from build123d import *

# Parameters (mm, degrees)
F0_R     = 3.175
F1_DEPTH = 3.048


with BuildPart() as f1:
    # F0 (on Front) → F1 (new body)
    with BuildSketch(Plane.XZ):
        with BuildLine():
            ThreePointArc((18.5272162363, -2.8907946242), (12.1944256202, -14.2446628188), (0, -18.7513848829))
            Line((0, -18.7513848829), (0, -51.0613519013))
            ThreePointArc((0, -51.0613519013), (6.7351920908, -53.8511598105), (9.525, -60.5863519013))
            Line((9.525, -60.5863519013), (36.5125, -60.5863519013))
            ThreePointArc((36.5125, -60.5863519013), (38.9380895153, -54.8747191174), (44.7324052746, -52.6538772867))
            Line((44.7324052746, -52.6538772867), (19.9038367454, -51.7699515192))
            ThreePointArc((19.9038367454, -51.7699515192), (14.056218392, -48.8866966862), (12.3315367458, -42.5991477155))
            Line((12.3315367458, -42.5991477155), (18.5272162363, -2.8907946242))
        make_face()
        with BuildLine():
            Line((36.5125, -60.5863519013), (9.525, -60.5863519013))
            ThreePointArc((9.525, -60.5863519013), (6.9705567315, -67.0776509895), (0.6773435479, -70.0872376873))
            Line((0.6773435479, -70.0872376873), (44.7324052746, -68.5188265159))
            ThreePointArc((44.7324052746, -68.5188265159), (38.9380895153, -66.2979846852), (36.5125, -60.5863519013))
        make_face()
        with BuildLine():
            Line((0, 18.7513848829), (0, 3.175))
            ThreePointArc((0, 3.175), (2.2450640303, 2.2450640303), (3.175, 0))
            ThreePointArc((3.175, 0), (2.2450640303, -2.2450640303), (0, -3.175))
            Line((0, -3.175), (0, -18.7513848829))
            ThreePointArc((0, -18.7513848829), (12.1944256202, -14.2446628188), (18.5272162363, -2.8907946242))
            ThreePointArc((18.5272162363, -2.8907946242), (18.6952587236, -1.4497366262), (18.7513848829, 0))
            ThreePointArc((18.7513848829, 0), (18.6943609499, 1.4612678406), (18.5236359763, 2.9136480987))
            Line((18.5236359763, 2.9136480987), (18.3973654955, 3.6264828487))
            ThreePointArc((18.3973654955, 3.6264828487), (11.9082504878, 14.4847507865), (0, 18.7513848829))
        make_face()
        with BuildLine():
            ThreePointArc((0, -3.175), (-3.175, 0), (0, 3.175))
            Line((0, 3.175), (0, 18.7513848829))
            ThreePointArc((0, 18.7513848829), (-12.0470149388, 14.3695464817), (-18.4637179825, 3.2719341818))
            ThreePointArc((-18.4637179825, 3.2719341818), (-18.7503896007, 0.1931963966), (-18.5272162363, -2.8907946242))
            ThreePointArc((-18.5272162363, -2.8907946242), (-12.1944256202, -14.2446628188), (0, -18.7513848829))
            Line((0, -18.7513848829), (0, -3.175))
        make_face()
        with BuildLine():
            Line((0, -57.4113519013), (0, -51.0613519013))
            ThreePointArc((0, -51.0613519013), (-6.7351920908, -53.8511598105), (-9.525, -60.5863519013))
            ThreePointArc((-9.525, -60.5863519013), (-6.7351920908, -67.3215439921), (0, -70.1113519013))
            Line((0, -70.1113519013), (0.6773435479, -70.0872376873))
            ThreePointArc((0.6773435479, -70.0872376873), (6.9705567315, -67.0776509895), (9.525, -60.5863519013))
            Line((9.525, -60.5863519013), (3.175, -60.5863519013))
            ThreePointArc((3.175, -60.5863519013), (-2.2450640303, -62.8314159316), (0, -57.4113519013))
        make_face()
        with BuildLine():
            ThreePointArc((9.525, -60.5863519013), (6.7351920908, -53.8511598105), (0, -51.0613519013))
            Line((0, -51.0613519013), (0, -57.4113519013))
            ThreePointArc((0, -57.4113519013), (2.2450640303, -58.341287871), (3.175, -60.5863519013))
            Line((3.175, -60.5863519013), (9.525, -60.5863519013))
        make_face()
        with BuildLine():
            ThreePointArc((-18.4637179825, 3.2719341818), (-12.0470149388, 14.3695464817), (0, 18.7513848829))
            Line((0, 18.7513848829), (0, 36.5252))
            Line((0, 36.5252), (0, 44.1886480987))
            ThreePointArc((0, 44.1886480987), (-6.7351920908, 46.9784560079), (-9.525, 53.7136480987))
            Line((-9.525, 53.7136480987), (-18.4637179825, 3.2719341818))
        make_face()
        with Locations((-3.175, 36.5252)):
            Circle(F0_R, mode=Mode.SUBTRACT)
        with BuildLine():
            Line((0, 36.5252), (0, 18.7513848829))
            ThreePointArc((0, 18.7513848829), (11.9082504878, 14.4847507865), (18.3973654955, 3.6264828487))
            Line((18.3973654955, 3.6264828487), (9.525, 53.7136480987))
            ThreePointArc((9.525, 53.7136480987), (6.7351920908, 46.9784560079), (0, 44.1886480987))
            Line((0, 44.1886480987), (0, 36.5252))
        make_face()
        with BuildLine():
            Line((0, -51.0613519013), (0, -18.7513848829))
            ThreePointArc((0, -18.7513848829), (-12.1944256202, -14.2446628188), (-18.5272162363, -2.8907946242))
            Line((-18.5272162363, -2.8907946242), (-9.525, -60.5863519013))
            ThreePointArc((-9.525, -60.5863519013), (-6.7351920908, -53.8511598105), (0, -51.0613519013))
        make_face()
        with BuildLine():
            ThreePointArc((44.7324052746, -52.6538772867), (38.9380895153, -54.8747191174), (36.5125, -60.5863519013))
            ThreePointArc((36.5125, -60.5863519013), (38.9380895153, -66.2979846852), (44.7324052746, -68.5188265159))
            ThreePointArc((44.7324052746, -68.5188265159), (50.1616327839, -66.098262386), (52.3875, -60.5863519013))
            ThreePointArc((52.3875, -60.5863519013), (50.1616327839, -55.0744414166), (44.7324052746, -52.6538772867))
        make_face()
        with BuildLine():
            ThreePointArc((47.625, -60.5863519013), (44.45, -63.7613519013), (41.275, -60.5863519013))
            ThreePointArc((41.275, -60.5863519013), (44.45, -57.4113519013), (47.625, -60.5863519013))
        make_face(mode=Mode.SUBTRACT)
        with BuildLine():
            ThreePointArc((-9.525, 53.7136480987), (-6.7351920908, 46.9784560079), (0, 44.1886480987))
            ThreePointArc((0, 44.1886480987), (6.7351920908, 46.9784560079), (9.525, 53.7136480987))
            ThreePointArc((9.525, 53.7136480987), (0, 63.2386480987), (-9.525, 53.7136480987))
        make_face()
        with BuildLine():
            ThreePointArc((3.175, 53.7136480987), (2.2450640303, 51.4685840684), (0, 50.5386480987))
            ThreePointArc((0, 50.5386480987), (-2.2450640303, 55.958712129), (3.175, 53.7136480987))
        make_face(mode=Mode.SUBTRACT)
    extrude(amount=F1_DEPTH)


solid = f1.part
The model under review builds one solid part; all positions refer to its coordinate system, in mm. Round coordinates to 2 decimals unless told otherwise and drop trailing zeros. Loops run counter-clockwise (first coordinate to the right, second up) from the corner with the lowest first, then second, coordinate; pieces in that order, holes last. Notation, with made-up numbers: M 49.25,14.25 L 66.25,14.25 A20 cw 66.25,43.25 Z; hole C 12.25,37 d6. An arc over 180 degrees is marked long. Answer as a JSON object with one key per item and string values.
Item 1: We need section C-C, the plane z = -54.5. State the section outline as (x, y) points.
Check sheet entries:
{"outline": "M -10.47,-3.05 L 49.55,-3.05 L 49.55,0 L -10.47,0 Z"}
Item 2: For line 1 along Z through (x, y) = (-2, -1.2); line 2 along Z through (x, y) = (44.45, -1.25); line 3 along Z through (x, y) = (38.5, -0.5), list the stretches that pass through material, from the lowest coordinate up.
Check sheet entries:
{"line 1": "-69.9 to -63.05, -58.12 to -2.47, 2.47 to 33.58, 39.47 to 51.25, 56.18 to 63.03", "line 2": "-68.53 to -63.76, -57.41 to -52.64", "line 3": "-68.74 to -52.43"}
Item 3: We need section A-A, the plane x = -5. State the section outline as (y, z) points, and give its area (3 significant figures).
Check sheet entries:
{"outline": "M -3.05,-68.69 L 0,-68.69 L 0,33.93 L -3.05,33.93 Z; M -3.05,39.12 L 0,39.12 L 0,61.82 L -3.05,61.82 Z", "area": "382 mm2"}
Item 4: Clearance check with flat-ended pins moving along their axes: P1, Ø1, axis at x = 30.5, y = -1.5, coming from the +Z side; P2, Ø1.5, axis at y = -1, z = -18.5, coming from the -X side. State where each tip first meets the part, or that it passes through.
Check sheet entries:
{"P1": "z = -52.13", "P2": "x = -16.21"}
Item 5: We need section B-B, the plane y = -1.85. State how many separate pieces and enclosed holes the cut face has, and give its area (3 significant figures).
Check sheet entries:
{"separate pieces": "1", "enclosed holes": "5", "area": "4,110 mm2"}
Item 6: We need section D-D, the plane x = 25.5. State the section outline as (y, z) points, and give its area (3 significant figures).
Check sheet entries:
{"outline": "M -3.05,-69.2 L 0,-69.2 L 0,-51.97 L -3.05,-51.97 Z", "area": "52.5 mm2"}
Item 7: The part is to be moulded in two halves that separate along X. For faces 1 (the face through (41.517, -1.503, -61.802)), 2 (the face through (-18.75, -1.5, 0.24)), 3 (the face through (8, 0, -17)), 4 (the face through (15.386, -1.503, -23.023)), say which applies: +X half, -X half, draft (parallel to the pull), parting line (faces both ways), or undercut.
Check sheet entries:
{"face 1": "undercut", "face 2": "-X half", "face 3": "draft", "face 4": "+X half"}
